Geometry check sheet. Reference: the model listing, model coordinates, mm. Face numbers are marked on the shaded views. A direction names the side the tool comes from. Round coordinates to 2 decimals unless told otherwise and drop trailing zeros. Write each loop counter-clockwise with the first axis right and the second up, starting at its lowest first coordinate (ties: lowest second). Pieces come first, ordered by that corner, then holes. Notation, with made-up numbers: M 29,-5 L 57,-5 A13 cw 57,16 Z; hole C 24,42.25 d9. An arc over 180 degrees is marked long. Put each result on its own line as item: value. Start each with the question number.
(1) Section check D-D on z = 2.75. Record the cut outline in (x, y), then the cut area to 3 significant figures.
(2) Tool access check on the marked faces 4 and 5. Record the directions out of +Z, -Z, +X, -X, +Y, -Y that give a thin tool (end or side, any length) a straight path to the whole face; none if there is none.
(3) Material ranges on probe 1 along Y at (x, z) = (27, 13.25); probe 2 along Z at (x, y) = (26.5, -5.5); probe 3 along X at (y, z) = (4.5, 16.5), recorded low to high.
(4) Mould release check, pull along X, two halves, no side actions. Record for the marked faces 1, 2 and 3: pulls with the +X half, pulls with the -X half, needs draft (parallel to the pull), parting line crosses it, or undercut.
(5) Gauge pin test, flat ends, axial feed: pin 1 (6 mm diameter, centred on x = 30.5, y = 7, fed in from -Z); pin 2 (10 mm diameter, centred on x = 5, z = 8.5, fed in from -Y); pin 3 (3 mm diameter, centred on y = 10, z = 11.5, fed in from +X). Record the tip position at first contact, or that the pin passes through.
(6) Section check A-A on z = 8.5. Record the cut outline in (x, y).
(7) Section check B-B on y = -1. Record the cut outline in (x, z), then the cut area to 3 significant figures.
(8) Section check C-C on x = -5.5. Record the cut outline in (y, z).
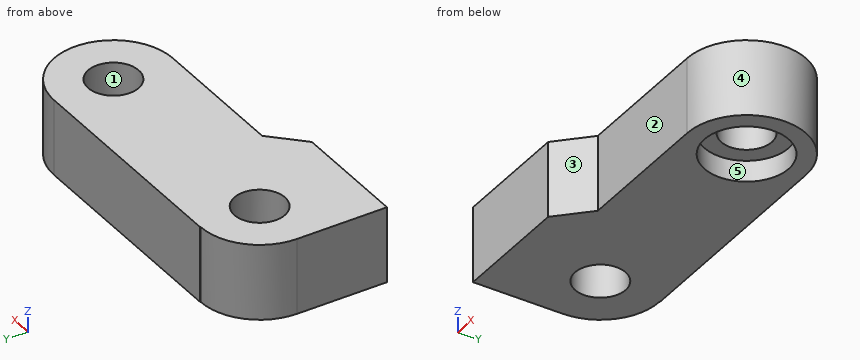
from build123d import *

# Parameters (mm, degrees)
SKETCH1_W           = 83
SKETCH1_H           = 35.4
SKETCH1_R           = 6
BOSS_EXTRUDE1_DEPTH = 18
CUT_EXTRUDE1_DEPTH  = 49.5750965
CUT_EXTRUDE2_DEPTH  = 49.5750965
SKETCH4_R           = 10
CUT_EXTRUDE3_DEPTH  = 5


with BuildPart() as part:
    # Sketch1 → Boss-Extrude1 (new body)
    with BuildSketch(Plane.XY):
        Rectangle(SKETCH1_W, SKETCH1_H)
        with Locations((-27.5, 3.6)):
            Circle(SKETCH1_R, mode=Mode.SUBTRACT)
        with Locations((27, 3.6)):
            Circle(SKETCH1_R, mode=Mode.SUBTRACT)
    extrude(amount=BOSS_EXTRUDE1_DEPTH)

    # Sketch2 → Cut-Extrude1 (cut, through all)
    with BuildSketch(Plane.XY.offset(18)):
        with BuildLine():
            Line((27, -10.5), (-6.3, -10.5))
            Line((-6.3, -10.5), (-13.5, -17.7))
            Line((-13.5, -17.7), (-41.5, -17.7))
            Line((-41.5, -17.7), (-41.5, -37.108146422))
            Line((-41.5, -37.108146422), (58.064931867, -37.108146422))
            Line((58.064931867, -37.108146422), (58.064931867, 31.4831893))
            Line((58.064931867, 31.4831893), (27, 31.4831893))
            Line((27, 31.4831893), (27, 17.7))
            ThreePointArc((27, 17.7), (41.1, 3.6), (27, -10.5))
        make_face()
    extrude(amount=-CUT_EXTRUDE1_DEPTH, mode=Mode.SUBTRACT)

    # Sketch3 → Cut-Extrude2 (cut, through all)
    with BuildSketch(Plane.XY.offset(18)):
        with BuildLine():
            Line((-27.5, 17.6), (-27.5, 27.141783499))
            Line((-27.5, 27.141783499), (-58.476255023, 27.141783499))
            Line((-58.476255023, 27.141783499), (-58.476255023, 3.6))
            Line((-58.476255023, 3.6), (-41.5, 3.6))
            ThreePointArc((-41.5, 3.6), (-37.399494937, 13.499494937), (-27.5, 17.6))
        make_face()
    extrude(amount=-CUT_EXTRUDE2_DEPTH, mode=Mode.SUBTRACT)

    # Sketch4 → Cut-Extrude3 (cut)
    with BuildSketch(Plane(origin=(0, 0, 0), x_dir=(-1, 0, 0), z_dir=(0, 0, -1))):
        with Locations((-27, 3.6)):
            Circle(SKETCH4_R)
    extrude(amount=-CUT_EXTRUDE3_DEPTH, mode=Mode.SUBTRACT)


solid = part.part
Answers follow:
1. outline: M -41.5,-17.7 L -13.5,-17.7 L -6.3,-10.5 L 27,-10.5 A14.1 ccw 27,17.7 L -27.5,17.7 L -27.5,17.6 A14 ccw -41.5,3.6 Z; hole C -27.5,3.6 d12; hole C 27,3.6 d20
1. area: 2,000 mm^2
2. face 4: +Z, -Z, +X
2. face 5: -Z
3. probe 1: y = -10.5 to -2.4, 9.6 to 17.7
3. probe 2: z = 5 to 18
3. probe 3: x = -41.47 to -33.43, -21.57 to 21.07, 32.93 to 41.07
4. face 1: undercut
4. face 2: needs draft
4. face 3: pulls with the +X half
5. pin 1: stops at z = 5
5. pin 2: stops at y = -10.5
5. pin 3: stops at x = 40.22
6. outline: M -41.5,-17.7 L -13.5,-17.7 L -6.3,-10.5 L 27,-10.5 A14.1 ccw 27,17.7 L -27.5,17.7 L -27.5,17.6 A14 ccw -41.5,3.6 Z; hole C -27.5,3.6 d12; hole C 27,3.6 d12
7. outline: M -41.5,0 L -31.35,0 L -31.35,18 L -41.5,18 Z; M -23.65,0 L 18.12,0 L 18.12,5 L 23.15,5 L 23.15,18 L -23.65,18 Z; M 30.85,5 L 35.88,5 L 35.88,0 L 40.33,0 L 40.33,18 L 30.85,18 Z
7. area: 1,150 mm^2
8. outline: M -10.5,0 L 17.7,0 L 17.7,18 L -10.5,18 Z
